The figure shows three views and two pictorial views of one solid part (mm, origin at its lowest corner). Answer the questions. A direction names the side the tool comes from. Round coordinates to 2 decimals unless told otherwise and drop trailing zeros. Order: outer loops, then holes, each group sorted by start corner. A loop starts at its lowest first (then second) coordinate and runs counter-clockwise, first axis right, second up. Notation, with made-up numbers: (-24.75, -16) - (20.25, -16) arc R20 ccw to (20.25, 19) - close; hole circle Ø10 at (70, -39.5). An arc over 180 degrees is marked (long way). Answer as a JSON object with one key per item and string values. Group by question number.
Q1. A cutting plane is placed at A-A on y = 22. Determine the outline of the cut face in (x, z) (1 decimal).
Q2. Consider line 1 (X direction, y = 16.75, z = 30.5); line 2 (Z direction, x = 5, y = 13) (1 decimal); line 3 (Z direction, x = 6.5, y = 20) (1 decimal). Determine where each line is inside the solid, lowest interval first.
Q3. Given pin 1 Ø4 at (y, z) = (13.5, 13.5) entering from -X, flat-ended and moving along its own axis, determine where the tip first touches the part or whether it passes through.
Q4. The mould has two halves that part along Z. Classify the marked faces 1, 2 and 3: pulls with the +Z half, pulls with the -Z half, needs draft (parallel to the pull), parting line crosses it, or undercut.
Q5. A cutting plane is placed at C-C on y = 17.5. Determine the outline of the cut face in (x, z), and give its area (3 significant figures).
Q6. A cutting plane is placed at B-B on z = 30. Determine the outline of the cut face in (x, y), and give its area (3 significant figures).
Q7. A cutting plane is placed at D-D on z = 45. Determine the outline of the cut face in (x, y), and give its area (3 significant figures).
Q8. A tool of negligible diameter and unlimited length cuts with its end or side. For the marked faces 4 and 5, from which of +Z, -Z, +X, -X, +Y, -Y can it reach the whole face along a straight path? Write none if from no direction.
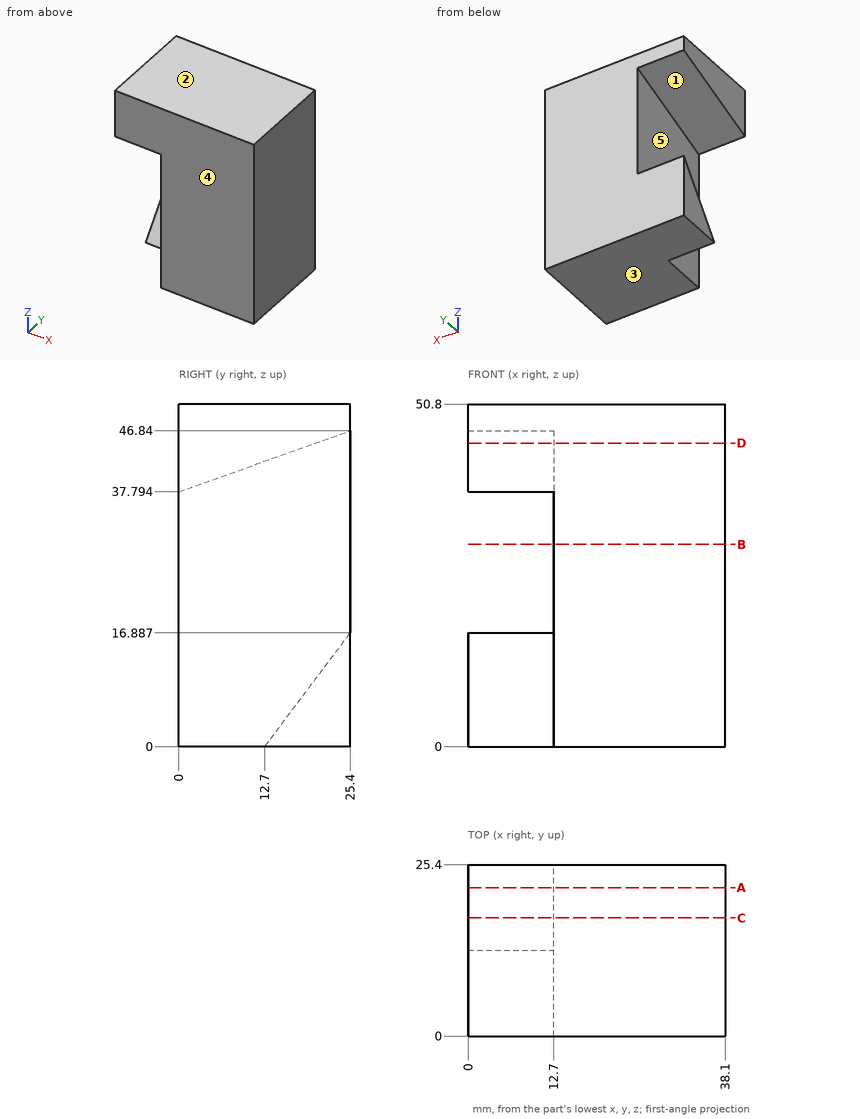
Result set:
{
 "1": {"outline": "(0, 0) - (38.1, 0) - (38.1, 50.8) - (0, 50.8) - (0, 45.6) - (12.7, 45.6) - (12.7, 12.4) - (0, 12.4) - close"},
 "2": {"line 1": "x = 12.7 to 38.1", "line 2": "z = 0 to 0.4, 42.4 to 50.8", "line 3": "z = 0 to 9.7, 44.9 to 50.8"},
 "3": {"pin 1": "stops at x = 12.7"},
 "4": {"face 1": "undercut", "face 2": "pulls with the +Z half", "face 3": "pulls with the -Z half"},
 "5": {"outline": "(0, 0) - (38.1, 0) - (38.1, 50.8) - (0, 50.8) - (0, 44.03) - (12.7, 44.03) - (12.7, 6.38) - (0, 6.38) - close", "area": "1,460 mm²"},
 "6": {"outline": "(12.7, 0) - (38.1, 0) - (38.1, 25.4) - (12.7, 25.4) - close", "area": "645 mm²"},
 "7": {"outline": "(0, 0) - (38.1, 0) - (38.1, 25.4) - (12.7, 25.4) - (12.7, 20.23) - (0, 20.23) - close", "area": "902 mm²"},
 "8": {"face 4": "+Z, -Z, +X, -X, -Y", "face 5": "-X"}
}
